from build123d import *

# Parameters (mm, degrees)
SKETCH_1_R          = 4
EXTRUDE_1_DEPTH     = 21
SKETCH_2_R          = 5
EXTRUDE_2_DEPTH     = 92
SKETCH_3_R          = 1.65
CUT_EXTRUDE_1_DEPTH = 20
CUT_EXTRUDE_START   = -5.3
SKETCH_7_R          = 5
SKETCH_7_R_2        = 3.95
CUT_EXTRUDE_4_DEPTH = 0.9
SKETCH_8_R          = 3
EXTRUDE_3_DEPTH     = 2.5
CHAMFER_1_SIZE      = 0.5
SKETCH_9_R          = 1.25
CUT_EXTRUDE_5_DEPTH = 7
CUT_EXTRUDE_START_2 = -3.3
SKETCH_7_2_R        = 5
SKETCH_7_2_R_2      = 3.95
CUT_EXTRUDE_6_DEPTH = 0.9


with BuildPart() as part:
    # 草图1 → 凸台-拉伸1 (new body)
    with BuildSketch(Plane(origin=(0, 0, 0), x_dir=(0, 0, -1), z_dir=(1, 0, 0))):
        with Locations(Location((0, 0, 0), (0, 0, 180))):
            Circle(SKETCH_1_R)
    extrude(amount=EXTRUDE_1_DEPTH)

    # 草图2 → 凸台-拉伸2 (add)
    with BuildSketch(Plane(origin=(21, 0, 0), x_dir=(0, 0, -1), z_dir=(1, 0, 0))):
        with Locations(Location((0, 0, 0), (0, 0, 270))):
            Circle(SKETCH_2_R)
    extrude(amount=EXTRUDE_2_DEPTH)

    # 草图3 → 切除-拉伸1 (cut)
    with BuildSketch(Plane(origin=(0, 7, 0), x_dir=(1, 0, 0), z_dir=(0, 1, 0))):
        with Locations(Location((3.5, 0, 0), (0, 0, 270))):
            Circle(SKETCH_3_R)
    extrude(amount=-CUT_EXTRUDE_1_DEPTH, mode=Mode.SUBTRACT)

    # 草图7 → 切除-拉伸4 (cut)
    with BuildSketch(Plane.ZY.offset(-101.5).offset(CUT_EXTRUDE_START)):
        with Locations(Location((0, 0, 0), (0, 0, 180))):
            Circle(SKETCH_7_R)
        with Locations(Location((0, 0, 0), (0, 0, 180))):
            Circle(SKETCH_7_R_2, mode=Mode.SUBTRACT)
    extrude(amount=-CUT_EXTRUDE_4_DEPTH, mode=Mode.SUBTRACT)

    # 草图8 → 凸台-拉伸3 (add)
    with BuildSketch(Plane(origin=(113, 0, 0), x_dir=(0, 0, -1), z_dir=(1, 0, 0))):
        Circle(SKETCH_8_R)
    extrude(amount=EXTRUDE_3_DEPTH)

    # 倒角1
    chamfer_1_edges = [part.edges().sort_by_distance(p)[0] for p in [
        (0, 0, -4),
        (115.5, 0, 3),
    ]]
    chamfer(chamfer_1_edges, length=CHAMFER_1_SIZE)

    # 草图9 → 切除-拉伸5 (cut)
    with BuildSketch(Plane(origin=(0, 5, 0), x_dir=(1, 0, 0), z_dir=(0, 1, 0))):
        with Locations(Location((81, 0, 0), (0, 0, 270))):
            Circle(SKETCH_9_R)
        with Locations(Location((53, 0, 0), (0, 0, 270))):
            Circle(SKETCH_9_R)
    extrude(amount=-CUT_EXTRUDE_5_DEPTH, mode=Mode.SUBTRACT)

    # 草图7<2> → 切除-拉伸6 (cut)
    with BuildSketch(Plane.ZY.offset(-101.5).offset(CUT_EXTRUDE_START_2)):
        with Locations(Location((0, 0, 0), (0, 0, 180))):
            Circle(SKETCH_7_2_R)
        with Locations(Location((0, 0, 0), (0, 0, 180))):
            Circle(SKETCH_7_2_R_2, mode=Mode.SUBTRACT)
    extrude(amount=CUT_EXTRUDE_6_DEPTH, mode=Mode.SUBTRACT)


solid = part.part
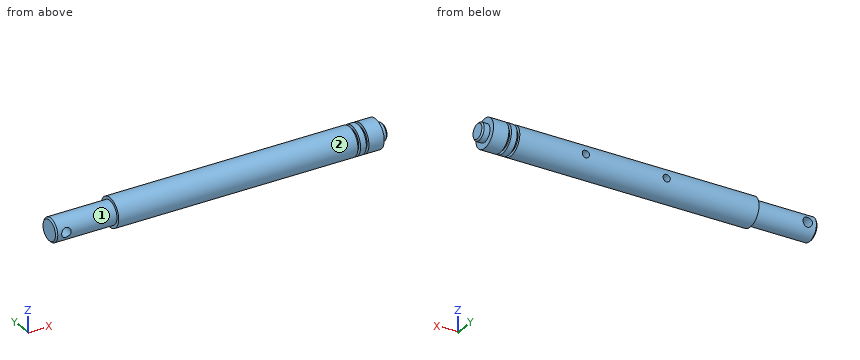
Here's how the part is built. I have some questions about the finished solid (model axes, mm). Face numbers are marked on the shaded views. A direction names the side the tool comes from. Give positions to 0.01 mm unless a question says otherwise; leave off trailing zeros. Loops run counter-clockwise (first coordinate to the right, second up) from the corner with the lowest first, then second, coordinate; pieces in that order, holes last. Notation, with made-up numbers: (-23, 31) -> (-10, 31) arc R17 cw to (-10, 64) -> close; hole circle Ø9 at (73, -15). An arc over 180 degrees is marked (long way). One line per item, written item: value.
Q1. Suppose I cut it at B-B on y = 0. State how many separate pieces and enclosed holes the cut face has, then the cut area to 3 significant figures.
Answers follow:
separate pieces: 1
enclosed holes: 3
area: 1,080 mm^2
Q2. I'm going to push flat-ended pins straight in: pin 1 Ø1 at (x, y) = (23.5, 4) entering from -Z; pin 2 Ø1 at (x, y) = (49, 1.5) entering from +Z; pin 3 Ø2 at (x, z) = (81, -0.5) entering from +Y. Where does each tip first touch, or does it pass through?
Answers follow:
pin 1: z = -3.57
pin 2: z = 4.9
pin 3: y = 4.93
Q3. Suppose I cut it at A-A on x = 3.5. Please give me the cut outline in (y, z), then the cut area to 3 significant figures.
Answers follow:
outline: (-3.64, -1.65) arc R4 ccw to (3.64, -1.65) -> close; (-3.64, 1.65) -> (3.64, 1.65) arc R4 ccw to start
area: 24.6 mm^2
Q4. If I drill on line 1 along X through (y, z) = (0.75, 0); line 2 along X through (y, z) = (-3.25, 3.75); line 3 along X through (y, z) = (3.75, 0), over which ranges is the centre line in solid material (lowest first)?
Answers follow:
line 1: 0 to 1.85, 5.15 to 51.75, 54.25 to 79.75, 82.25 to 115.5
line 2: 21 to 103.9, 104.8 to 106.8, 107.7 to 113
line 3: 0.25 to 1.85, 5.15 to 51.75, 54.25 to 79.75, 82.25 to 113
Q5. Suppose I cut it at C-C on x = 64. Please give me the cut outline in (y, z).
Answers follow:
outline: circle Ø10 at (0, 0)
Q6. On a 3-axis mill with a long thin cutter (end or side, diameter ignored), from which of +Z, -Z, +X, -X, +Y, -Y can I reach the whole of each face in a straight line? I mean the marked faces 1 and 2. Say none if no direction works.
Answers follow:
face 1: -X
face 2: +X, -X
